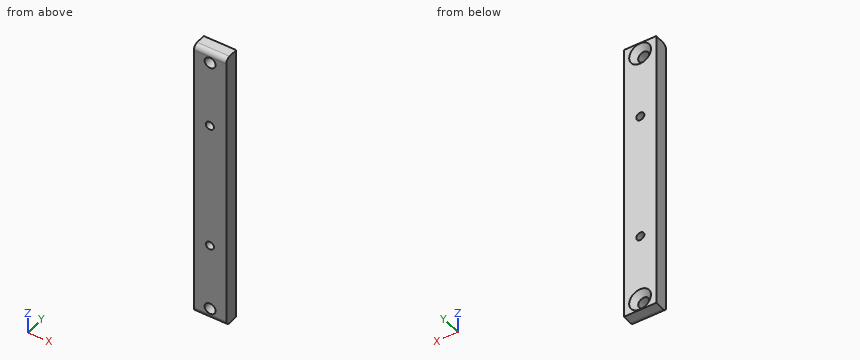
```python
from build123d import *

# Parameters (mm, degrees)
SKETCH1_W                                            = 89
SKETCH1_H                                            = 4.5
BOSS_EXTRUDE1_DEPTH                                  = 10
FILLET1_R                                            = 1.5
CSK_FOR_M3_HEX_SOCKET_COUNTERSUNK_CAP_SC_D           = 3.4
CSK_FOR_M3_HEX_SOCKET_COUNTERSUNK_CAP_SC_CSINK_D     = 6.72
CSK_FOR_M3_HEX_SOCKET_COUNTERSUNK_CAP_SC_CSINK_ANGLE = 90
M3_TAPPED_HOLE1_D                                    = 2.5
M3_TAPPED_HOLE1_DEPTH                                = 7.5
M3_TAPPED_HOLE1_TIP                                  = 0.751075774


with BuildPart() as part:
    # Sketch1 → Boss-Extrude1 (new body)
    with BuildSketch(Plane(origin=(0, 0, 0), x_dir=(0, 0, -1), z_dir=(1, 0, 0))):
        with Locations((44.5, -2.25)):
            Rectangle(SKETCH1_W, SKETCH1_H)
    extrude(amount=BOSS_EXTRUDE1_DEPTH)

    # Fillet1
    fillet1_edges = [part.edges().sort_by_distance(p)[0] for p in [
        (5, -4.5, -89),
        (5, -4.5, 0),
    ]]
    fillet(fillet1_edges, radius=FILLET1_R)

    # CSK for M3 Hex Socket Countersunk Cap Screw1 (through all)
    with Locations(Plane(origin=(0, 0, 0), x_dir=(1, 0, 0), z_dir=(0, 1, 0))):
        with Locations((5, 3.5), (5, 85.5)):
            CounterSinkHole(CSK_FOR_M3_HEX_SOCKET_COUNTERSUNK_CAP_SC_D / 2, CSK_FOR_M3_HEX_SOCKET_COUNTERSUNK_CAP_SC_CSINK_D / 2, counter_sink_angle=CSK_FOR_M3_HEX_SOCKET_COUNTERSUNK_CAP_SC_CSINK_ANGLE)

    # M3 Tapped Hole1
    with Locations(Plane(origin=(0, 0, 0), x_dir=(1, 0, 0), z_dir=(0, 1, 0))):
        with Locations((4.933736509, 24.5), (4.933736509, 64.5)):
            Hole(M3_TAPPED_HOLE1_D / 2, depth=M3_TAPPED_HOLE1_DEPTH)
            with Locations((0, 0, -(M3_TAPPED_HOLE1_DEPTH + M3_TAPPED_HOLE1_TIP / 2))):  # 118° drill point
                Cone(0, M3_TAPPED_HOLE1_D / 2, M3_TAPPED_HOLE1_TIP, mode=Mode.SUBTRACT)


solid = part.part
```
Part model, mm, in its own coordinate system. Round coordinates to 2 decimals unless told otherwise and drop trailing zeros. Loops run counter-clockwise (first coordinate to the right, second up) from the corner with the lowest first, then second, coordinate; pieces in that order, holes last.
Item 1: Cut at A-A, the plane z = -85.5. Give the cut face in (x, y).
Item 2: Drop a flat-ended pin along its axis: P1, Ø4.5, axis at x = 5, z = -3.5, coming from the +Y side. Give the stop position or say it passes through.
Item 3: Cut at B-B, the plane x = 5. Give the cut face in (y, z), then the cut area to 3 significant figures.
Item 4: Drill centre lines: line 1 (Z direction, x = 5, y = -3.65); line 2 (X direction, y = -2.6, z = -85.5); line 3 (X direction, y = -2.5, z = -24.5). Where is each one in solid material? Low to high.
Item 5: Cut at C-C, the plane y = -3.7. Give the cut face in (x, z), then the cut area to 3 significant figures.
Item 6: Cut at D-D, the plane z = -64.5. Give the cut face in (x, y), then the cut area to 4 significant figures.
A:
1. outline: (0, -4.5) - (3.3, -4.5) - (3.3, -1.66) - (1.64, 0) - (0, 0) - close; (6.7, -4.5) - (10, -4.5) - (10, 0) - (8.36, 0) - (6.7, -1.66) - close
2. P1: stops at y = -1.11
3. outline: (-4.5, -87.5) arc R1.5 ccw to (-3, -89) - (0, -89) - (0, -88.86) - (-1.66, -87.2) - (-4.5, -87.2) - close; (-4.5, -83.8) - (-1.66, -83.8) - (0, -82.14) - (0, -65.75) - (-4.5, -65.75) - close; (-4.5, -63.25) - (0, -63.25) - (0, -25.75) - (-4.5, -25.75) - close; (-4.5, -23.25) - (0, -23.25) - (0, -6.86) - (-1.66, -5.2) - (-4.5, -5.2) - close; (-4.5, -1.8) - (-1.66, -1.8) - (0, -0.14) - (0, 0) - (-3, 0) arc R1.5 ccw to (-4.5, -1.5) - close
3. area: 341 mm2
4. line 1: z = -88.85 to -87.2, -83.8 to -65.75, -63.25 to -25.75, -23.25 to -5.2, -1.8 to -0.15
4. line 2: x = 0 to 3.3, 6.7 to 10
4. line 3: x = 0 to 3.68, 6.18 to 10
5. outline: (0, -88.83) - (10, -88.83) - (10, -0.17) - (0, -0.17) - close; hole circle Ø3.4 at (5, -85.5); hole circle Ø3.4 at (5, -3.5); hole circle Ø2.5 at (4.93, -64.5); hole circle Ø2.5 at (4.93, -24.5)
5. area: 859 mm2
6. outline: (0, -4.5) - (3.68, -4.5) - (3.68, 0) - (0, 0) - close; (6.18, -4.5) - (10, -4.5) - (10, 0) - (6.18, 0) - close
6. area: 33.75 mm2
